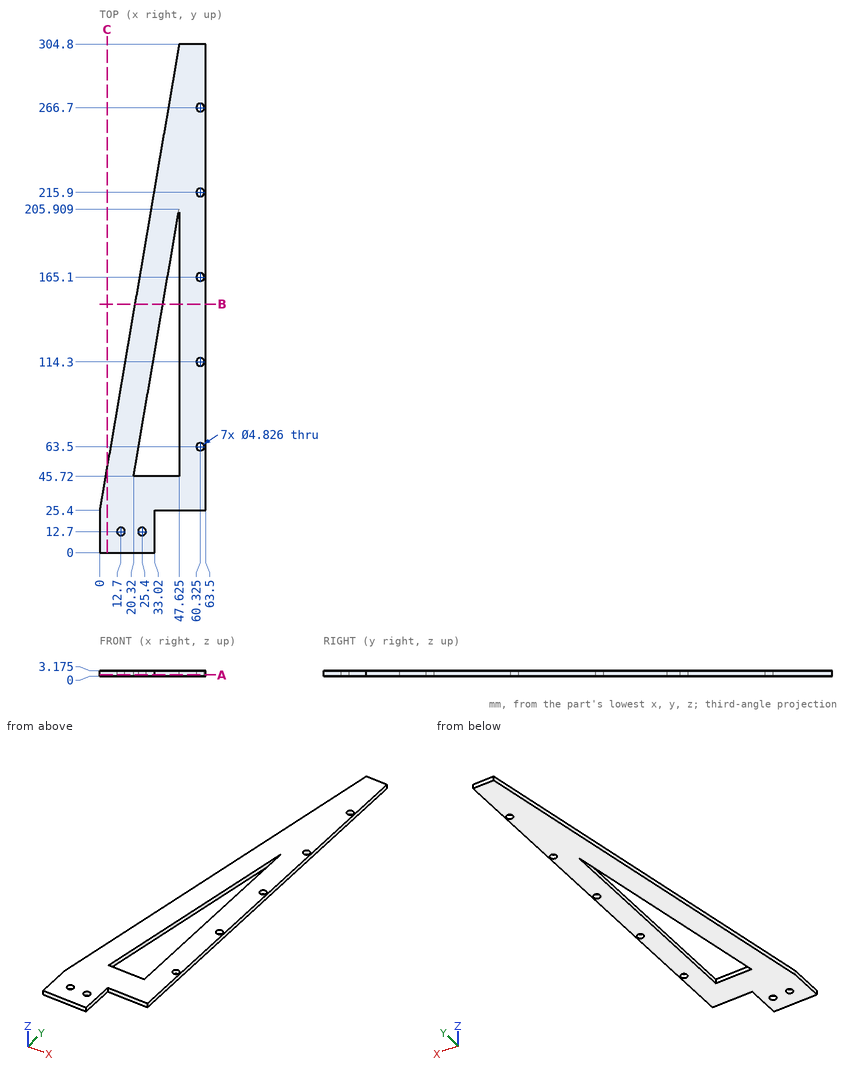
Print and shaded views of the part. All mm, measured from the part's lowest x, y and z. Give positions to 0.01 mm unless a question says otherwise; leave off trailing zeros. Loops run counter-clockwise (first coordinate to the right, second up) from the corner with the lowest first, then second, coordinate; pieces in that order, holes last. Notation, with made-up numbers: (38, 44) - (71, 44) arc R25 cw to (71, 80) - close; hole circle Ø8 at (44, -34). An arc over 180 degrees is marked (long way). One line per item, written item: value. Start each with the question number.
1. Slice it at B-B (y = 149). List the corners of the cut face in (x, z) (1 decimal).
2. Slice it at A-A (z = 0.6). Give the number of separate pieces and of enclosed holes in the cut face, plus the area to 3 significant figures.
3. Slice it at C-C (x = 4.5). List the corners of the cut face in (y, z) (1 decimal).
4. Pin check, flat tips, straight feed: pin 1 (3 mm diameter, centred on x = 60.325, y = 63.5, fed in from +Z); pin 2 (1.6 mm diameter, centred on y = 116, z = 1.5, fed in from -X). Stop position of each tip, or through.
5. Probe L1, parallel to X at y = 115, z = 2.55 (1 decimal); L2, parallel to Y at x = 48, z = 2.9; L3, parallel to X at y = 96, z = 2.45 (1 decimal). List the from-to ranges inside material, lowest first. Write a range as from..to.
Solution:
1. outline: (21.1, 0) - (37.9, 0) - (37.9, 3.2) - (21.1, 3.2) - close; (47.6, 0) - (63.5, 0) - (63.5, 3.2) - (47.6, 3.2) - close
2. separate pieces: 1
2. enclosed holes: 8
2. area: 9,610 mm^2
3. outline: (0, 0) - (51.8, 0) - (51.8, 3.2) - (0, 3.2) - close
4. pin 1: passes through
4. pin 2: stops at x = 15.31
5. L1: x = 15.3..32.1, 47.6..58, 62.6..63.5
5. L2: y = 25.4..304.8
5. L3: x = 12..28.9, 47.6..63.5
